Part print with two shaded views. Sizes in mm from the minimum x, y, z corner. A direction names the side the tool comes from. Round coordinates to 2 decimals unless told otherwise and drop trailing zeros. Write each loop counter-clockwise with the first axis right and the second up, starting at its lowest first coordinate (ties: lowest second). Pieces come first, ordered by that corner, then holes. Notation, with made-up numbers: M 68,37 L 122,37 A15 cw 122,50 Z; hole C 41.25,8 d7. An arc over 180 degrees is marked long. Use one line per item in the form item = value. Start each with the question number.
Item 1: Mould opens along Y. For the marked faces 1, 2 and 3 say: +Y half, -Y half, draft (parallel to the pull), parting line (faces both ways), or undercut.
Item 2: Cut at B-B, the plane x = 34. Give the cut face in (y, z) (1 decimal).
Item 3: Cut at A-A, the plane y = 26. Give the cut face in (x, z) (1 decimal).
Item 4: Cut at D-D, the plane x = 6. Give the cut face in (y, z), then the cut area to 3 significant figures.
Item 5: Probe L1, parallel to Y at x = 29.5, z = 2.5; L2, parallel to X at y = 43.5, z = 5.5 (1 decimal); L3, parallel to X at y = 15.5, z = 7 (1 decimal). List the from-to ranges inside material, lowest first.
Item 6: Which spindle directions (+Z, -Z, +X, -X, +Y, -Y) get a long thin tool onto all of the face, cutting with end or side? Do the marked faces 4, 5 and 6. Say none if no direction does.
Item 7: Flat gauge pin, fed straight in: pin 1 Ø1 at (x, z) = (12, 4.5) entering from -Y (1 decimal). Where does the tip first touch, or does it go through?
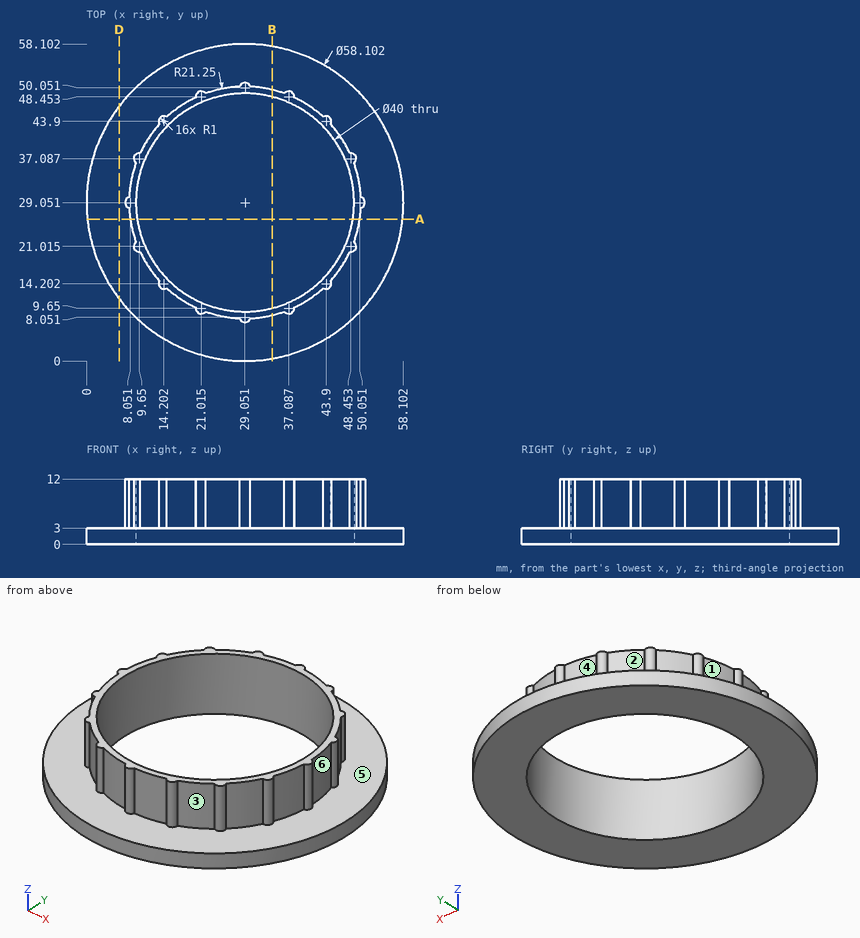
Model answer:
q1.face_1 = undercut
q1.face_2 = +Y half
q1.face_3 = -Y half
q2.outline = M 0.4,0 L 9.7,0 L 9.7,12 L 8.4,12 L 8.4,3 L 0.4,3 Z; M 48.4,0 L 57.7,0 L 57.7,3 L 49.7,3 L 49.7,12 L 48.4,12 Z
q3.outline = M 0.2,0 L 9.3,0 L 9.3,12 L 8,12 L 8,3 L 0.2,3 Z; M 48.8,0 L 57.9,0 L 57.9,3 L 50.1,3 L 50.1,12 L 48.8,12 Z
q4.outline = M 11.37,0 L 46.73,0 L 46.73,3 L 11.37,3 Z
q4.area = 106 mm²
q5.L1 = 0 to 9.06, 49.05 to 58.1
q5.L2 = 13.3 to 15.2, 42.9 to 44.8
q5.L3 = 12.7 to 14.3, 43.8 to 45.4
q6.face_4 = +Z, +Y
q6.face_5 = +Z
q6.face_6 = +Z, +X
q7.pin_1 = 15.7
